For this review, use the dimensioned drawing (mm, ordinates from the lowest corner) and the shaded views. Coordinates: 2 decimals unless noted, no trailing zeros. Loops run counter-clockwise (first coordinate to the right, second up) from the corner with the lowest first, then second, coordinate; pieces in that order, holes last.
1. Take a section at A-A, the plane y = 16. State the section outline as (x, z) points.
2. To check wall thickness, follow probe 1 along X at (y, z) = (27, 27); probe 2 along Y at (x, z) = (10, 20.5). State the ranges of each line that lie inside material, in increasing order.
3. Take a section at C-C, the plane x = 6.5. State the section outline as (y, z) points, then the cut area to 3 significant figures.
4. Clearance check with flat-ended pins moving along their axes: P1, Ø1, axis at x = 9.5, y = 5, coming from the +Z side; P2, Ø4, axis at x = 2, z = 10.5, coming from the -Y side; P3, Ø4, axis at x = 5.5, z = 27, coming from the -Y side. State where each tip first meets the part, or that it passes through.
5. Take a section at D-D, the plane y = 24. State the section outline as (x, z) points.
6. Mouldability with a two-part tool opening along X and no side actions: class the marked faces 1, 2, 3 and 4 as pulls with the +X half, pulls with the -X half, needs draft (parallel to the pull), parting line crosses it, or undercut.
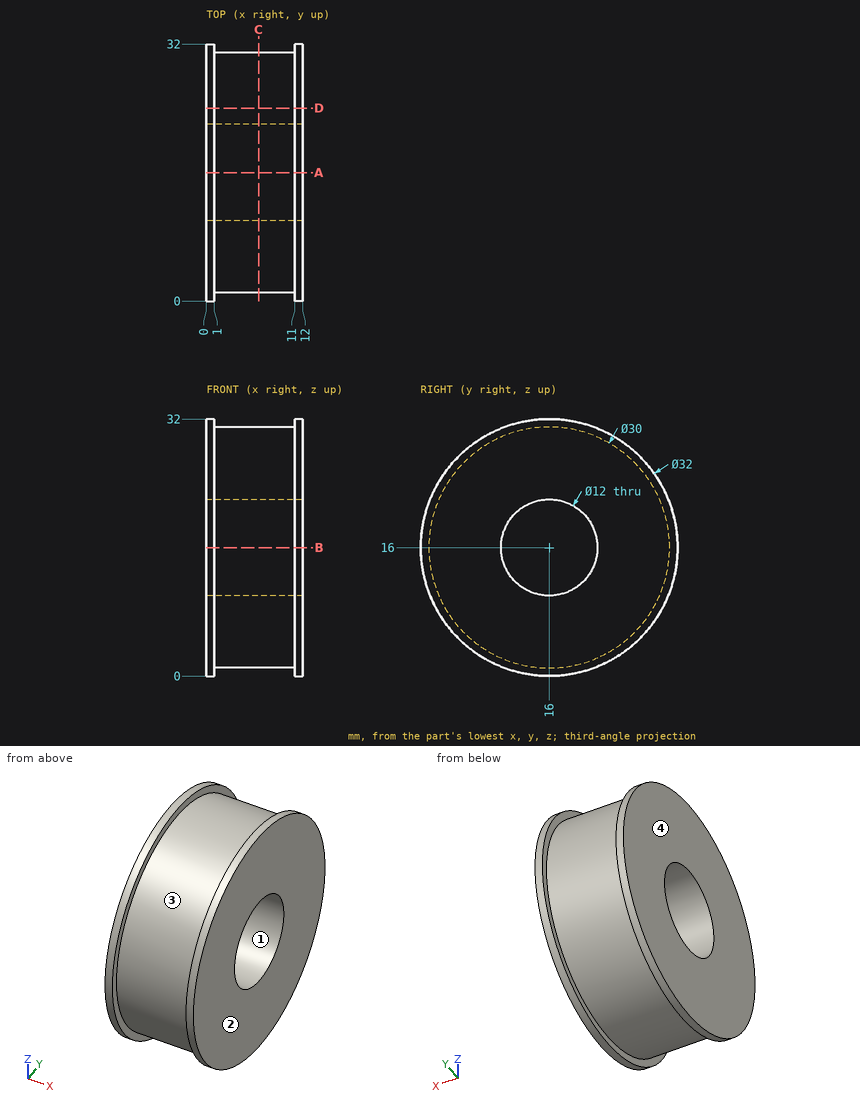
Results list:
1. outline: (0, 0) - (1, 0) - (1, 1) - (11, 1) - (11, 0) - (12, 0) - (12, 10) - (0, 10) - close; (0, 22) - (12, 22) - (12, 32) - (11, 32) - (11, 31) - (1, 31) - (1, 32) - (0, 32) - close
2. probe 1: x = 0 to 1, 11 to 12
2. probe 2: y = 1.69 to 12.03, 19.97 to 30.31
3. outline: circle Ø30 at (16, 16); hole circle Ø12 at (16, 16)
3. area: 594 mm2
4. P1: stops at z = 26.71
4. P2: stops at y = 0.45
4. P3: stops at y = 4
5. outline: (0, 2.14) - (1, 2.14) - (1, 3.31) - (11, 3.31) - (11, 2.14) - (12, 2.14) - (12, 29.86) - (11, 29.86) - (11, 28.69) - (1, 28.69) - (1, 29.86) - (0, 29.86) - close
6. face 1: needs draft
6. face 2: pulls with the +X half
6. face 3: undercut
6. face 4: pulls with the -X half
